Build history of the part. All positions in model axes, mm. Face numbers are marked on the shaded views. A direction names the side the tool comes from. Give positions to 0.01 mm unless a question says otherwise; leave off trailing zeros. Order: outer loops, then holes, each group sorted by start corner. A loop starts at its lowest first (then second) coordinate and runs counter-clockwise, first axis right, second up. Notation, with made-up numbers: (-2.75, 8) -> (38.25, 8) arc R20 ccw to (38.25, 24) -> close; hole circle Ø11 at (14, 26). An arc over 180 degrees is marked (long way). Write item = value, one per line. Start each with the question number.
from build123d import *

# Parameters (mm, degrees)
SKETCH008_W              = 40
SKETCH008_H              = 20
SKETCH008_R              = 2.75
PAD005_DEPTH             = 6
SKETCH009_W              = 18
SKETCH009_H              = 20
PAD006_DEPTH             = 26.8
SKETCH010_R              = 4
POCKET001_DEPTH          = 20.001
SKETCH011_W              = 2
SKETCH011_H              = 8.8415096984
POCKET002_DEPTH          = 20.001
SKETCH012_R              = 2.2
POCKET003_DEPTH          = 29.001
CLONE011_PLACEMENT_ANGLE = 90


with BuildPart() as part:
    # Sketch008 → Pad005 (new body)
    with BuildSketch(Plane.XY):
        Rectangle(SKETCH008_W, SKETCH008_H)
        with Locations((-16, 0)):
            Circle(SKETCH008_R, mode=Mode.SUBTRACT)
        with Locations((16, 0)):
            Circle(SKETCH008_R, mode=Mode.SUBTRACT)
    extrude(amount=PAD005_DEPTH)

    # Sketch009 (on Face8 of Pad005) → Pad006 (join)
    with BuildSketch(Plane.XY.offset(6)):
        Rectangle(SKETCH009_W, SKETCH009_H)
    extrude(amount=PAD006_DEPTH)

    # Sketch010 (on Face14 of Pad006) → Pocket001 (cut, through all)
    with BuildSketch(Plane.XZ.offset(10)):
        with Locations((0, 20)):
            Circle(SKETCH010_R)
    extrude(amount=-POCKET001_DEPTH, mode=Mode.SUBTRACT)

    # Sketch011 (on Face15 of Pocket001) → Pocket002 (cut, through all)
    with BuildSketch(Plane.XZ.offset(10)):
        with Locations((0, 28.3792451508)):
            Rectangle(SKETCH011_W, SKETCH011_H)
    extrude(amount=-POCKET002_DEPTH, mode=Mode.SUBTRACT)

    # Sketch012 (on Face12 of Pocket002) → Pocket003 (cut, through all)
    with BuildSketch(Plane.YZ.offset(9)):
        with Locations((0, 30)):
            Circle(SKETCH012_R)
    extrude(amount=-POCKET003_DEPTH, mode=Mode.SUBTRACT)


with BuildPart() as part_1:
    # Clone011 placement: moved
    add(part.part.moved(Location((10, -100, 10))).rotate(Axis((10, -100, 10), (0, 0, 1)), CLONE011_PLACEMENT_ANGLE))


solid = part_1.part
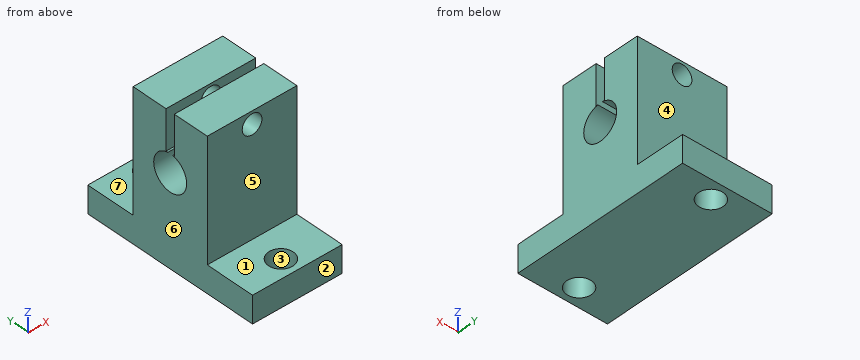
(1) Cut at D-D, the plane y = -103.5. Give the cut face in (x, z).
(2) 3-axis set-ups, long thin cutter, end or side, ignore diameter. For the marked faces 5, 6 and 7: which of +Z, -Z, +X, -X, +Y, -Y reach the whole face in a straight line?
(3) Cut at B-B, the plane z = 40. Give the cut face in (x, y), plus the area to 3 significant figures.
(4) Mould opens along Y. For the marked faces 1, 2, 3 and 4 say: released by +Y, released by -Y, zero draft, split by the parting line, or undercut.
(5) Cut at A-A, the plane y = -84. Give the cut face in (x, z).
(6) Flat gauge pins, fed straight in: P1, Ø5, axis at x = 10, z = 40, coming from the +Y side; P2, Ø12, axis at x = 12, y = -84, coming from the +Z side; P3, Ø4.5, axis at x = 6, z = 37, coming from the -Y side. Where does each tip first touch, or does it go through?
(7) Cut at C-C, the plane z = 30. Give the cut face in (x, y), plus the area to 3 significant figures.
(8) Wall check: line 1 (X direction, y = -116, z = 13); line 2 (Y direction, x = 6, z = 34.5); line 3 (Y direction, x = 13.75, z = 30). Give the ranges that are in metal, low to high. Write a range as [from, to].
Results:
q1.outline = (0, 10) -> (20, 10) -> (20, 28.06) -> (0, 28.06) -> close; (0, 31.94) -> (20, 31.94) -> (20, 42.8) -> (0, 42.8) -> close; hole circle Ø4.4 at (10, 40)
q2.face_5 = +Z, +X, -X, -Y
q2.face_6 = +Z, -Z, -X, +Y, -Y
q2.face_7 = +Z, +X, -X, +Y
q3.outline = (0, -109) -> (7.8, -109) -> (7.8, -101) -> (0, -101) -> close; (0, -99) -> (7.8, -99) -> (7.8, -91) -> (0, -91) -> close; (12.2, -109) -> (20, -109) -> (20, -101) -> (12.2, -101) -> close; (12.2, -99) -> (20, -99) -> (20, -91) -> (12.2, -91) -> close
q3.area = 250 mm2
q4.face_1 = zero draft
q4.face_2 = released by -Y
q4.face_3 = undercut
q4.face_4 = released by +Y
q5.outline = (0, 10) -> (7.25, 10) -> (7.25, 16) -> (0, 16) -> close; (12.75, 10) -> (20, 10) -> (20, 16) -> (12.75, 16) -> close
q6.P1 = -91
q6.P2 = 16
q6.P3 = -109
q7.outline = (0, -109) -> (20, -109) -> (20, -104) -> (0, -104) -> close; (0, -96) -> (20, -96) -> (20, -91) -> (0, -91) -> close
q7.area = 200 mm2
q8.line_1 = [0, 7.25], [12.75, 20]
q8.line_2 = [-109, -101], [-99, -91]
q8.line_3 = [-109, -104], [-96, -91]
